```python
from build123d import *

# Parameters (mm, degrees)
SKETCH015_W                     = 86
SKETCH015_H                     = 175
PAD007_DEPTH                    = 40
SKETCH016_W                     = 84
SKETCH016_H                     = 173
POCKET007_DEPTH                 = 38
SKETCH017_W                     = 23
SKETCH017_H                     = 14
PAD008_DEPTH                    = 20
SKETCH017_LINEARPATTERN003_2_W  = 23
SKETCH017_LINEARPATTERN003_2_H  = 14
PAD008_LINEARPATTERN003_2_DEPTH = 20
SKETCH017_LINEARPATTERN003_3_W  = 23
SKETCH017_LINEARPATTERN003_3_H  = 14
PAD008_LINEARPATTERN003_3_DEPTH = 20
SKETCH017_LINEARPATTERN003_4_W  = 23
SKETCH017_LINEARPATTERN003_4_H  = 14
PAD008_LINEARPATTERN003_4_DEPTH = 20
SKETCH017_LINEARPATTERN003_5_W  = 23
SKETCH017_LINEARPATTERN003_5_H  = 14
PAD008_LINEARPATTERN003_5_DEPTH = 20
LINEARPATTERN004_COUNT          = 2
LINEARPATTERN004_PITCH          = 28
FILLET008_R                     = 5
FILLET009_R                     = 2


with BuildPart() as part:
    # Sketch015 → Pad007 (new body)
    with BuildSketch(Plane.XY):
        Rectangle(SKETCH015_W, SKETCH015_H)
    extrude(amount=PAD007_DEPTH)

    # Sketch016 (on DatumPlane) → Pocket007 (cut)
    with BuildSketch(Plane.XY.offset(40)):
        Rectangle(SKETCH016_W, SKETCH016_H)
    extrude(amount=-POCKET007_DEPTH, mode=Mode.SUBTRACT)

    # Sketch017 (on DatumPlane) → Pad008 (join)
    with BuildSketch(Plane(origin=(-20, 65, 2), x_dir=(1, 0, 0), z_dir=(0, 0, 1))):
        Rectangle(SKETCH017_W, SKETCH017_H)
    pad008 = extrude(amount=PAD008_DEPTH)

    # Sketch017 LinearPattern003 2 → Pad008 LinearPattern003 2 (add)
    with BuildSketch(Plane(origin=(-20, 32.5, 2), x_dir=(1, 0, 0), z_dir=(0, 0, 1))):
        Rectangle(SKETCH017_LINEARPATTERN003_2_W, SKETCH017_LINEARPATTERN003_2_H)
    pad008_linearpattern003_2 = extrude(amount=PAD008_LINEARPATTERN003_2_DEPTH)

    # Sketch017 LinearPattern003 3 → Pad008 LinearPattern003 3 (add)
    with BuildSketch(Plane(origin=(-20, 0, 2), x_dir=(1, 0, 0), z_dir=(0, 0, 1))):
        Rectangle(SKETCH017_LINEARPATTERN003_3_W, SKETCH017_LINEARPATTERN003_3_H)
    pad008_linearpattern003_3 = extrude(amount=PAD008_LINEARPATTERN003_3_DEPTH)

    # Sketch017 LinearPattern003 4 → Pad008 LinearPattern003 4 (add)
    with BuildSketch(Plane(origin=(-20, -32.5, 2), x_dir=(1, 0, 0), z_dir=(0, 0, 1))):
        Rectangle(SKETCH017_LINEARPATTERN003_4_W, SKETCH017_LINEARPATTERN003_4_H)
    pad008_linearpattern003_4 = extrude(amount=PAD008_LINEARPATTERN003_4_DEPTH)

    # Sketch017 LinearPattern003 5 → Pad008 LinearPattern003 5 (add)
    with BuildSketch(Plane(origin=(-20, -65, 2), x_dir=(1, 0, 0), z_dir=(0, 0, 1))):
        Rectangle(SKETCH017_LINEARPATTERN003_5_W, SKETCH017_LINEARPATTERN003_5_H)
    pad008_linearpattern003_5 = extrude(amount=PAD008_LINEARPATTERN003_5_DEPTH)

    # LinearPattern004: Pad008, Pad008 LinearPattern003 2, Pad008 LinearPattern003 3, Pad008 LinearPattern003 4, Pad008 LinearPattern003 5 ×2
    with Locations(*[(i * LINEARPATTERN004_PITCH, 0, 0) for i in range(1, LINEARPATTERN004_COUNT)]):
        add(pad008)
        add(pad008_linearpattern003_2)
        add(pad008_linearpattern003_3)
        add(pad008_linearpattern003_4)
        add(pad008_linearpattern003_5)

    # Fillet008
    fillet008_edges = [part.edges().sort_by_distance(p)[0] for p in [
        (-20, -25.5, 22),
        (-8.5, -32.5, 22),
        (-20, -39.5, 22),
        (-31.5, -32.5, 22),
        (-20, -58, 22),
        (-8.5, -65, 22),
        (-20, -72, 22),
        (-31.5, -65, 22),
        (8, -58, 22),
        (19.5, -65, 22),
        (8, -72, 22),
        (-3.5, -65, 22),
        (8, -25.5, 22),
        (19.5, -32.5, 22),
        (8, -39.5, 22),
        (-3.5, -32.5, 22),
        (-20, 7, 22),
        (-8.5, 0, 22),
        (-20, -7, 22),
        (-31.5, 0, 22),
        (8, 7, 22),
        (19.5, 0, 22),
        (8, -7, 22),
        (-3.5, 0, 22),
        (8, 39.5, 22),
        (19.5, 32.5, 22),
        (8, 25.5, 22),
        (-3.5, 32.5, 22),
        (-20, 72, 22),
        (-8.5, 65, 22),
        (-20, 58, 22),
        (-31.5, 65, 22),
        (8, 72, 22),
        (19.5, 65, 22),
        (8, 58, 22),
        (-3.5, 65, 22),
        (-20, 39.5, 22),
        (-8.5, 32.5, 22),
        (-20, 25.5, 22),
        (-31.5, 32.5, 22),
    ]]
    fillet(fillet008_edges, radius=FILLET008_R)

    # Fillet009
    fillet009_edges = [part.edges().sort_by_distance(p)[0] for p in [
        (0, 87.5, 0),
        (43, 0, 0),
        (0, -87.5, 0),
        (-43, 0, 0),
    ]]
    fillet(fillet009_edges, radius=FILLET009_R)


with BuildPart() as part_1:
    # Body006 placement: moved
    add(part.part.moved(Location((-51, -51, 0))))


solid = part_1.part
```
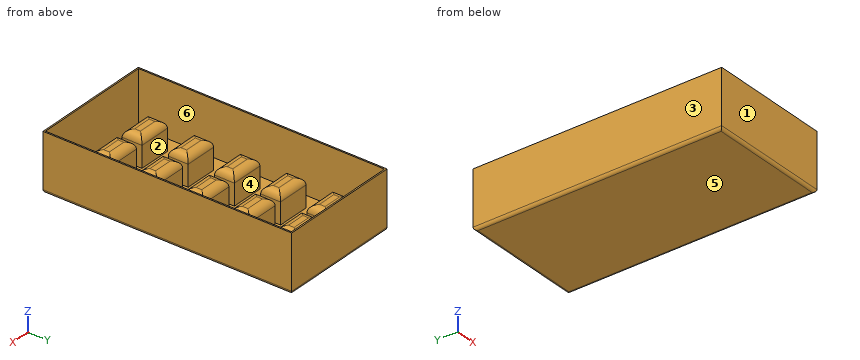
Check sheet for the modelled part. Datum: model origin and axes. Units: mm. Face numbers are marked on the shaded views. A direction names the side the tool comes from. Give positions to 0.01 mm unless a question says otherwise; leave off trailing zeros. Write each loop counter-clockwise with the first axis right and the second up, starting at its lowest first coordinate (ties: lowest second). Pieces come first, ordered by that corner, then holes.
Item 1: Draft check along X on the marked faces 3, 4, 5 and 6. Enter one of: released by +X, released by -X, zero draft, split by the parting line, or undercut.
Item 2: Scan lines: L1, parallel to X at y = -85, z = 37.5; L2, parallel to Y at x = -29, z = 31.5; L3, parallel to Z at x = -33.5, y = -126. Record each from-to range of solid material in increasing order.
Item 3: Cross-section at D-D (z = 35). Enter the section's corners in (x, y).
Item 4: Cross-section at A-A (z = 7.5). Count the separate pieces of the cut face and the enclosed holes in it, and give its area (3 significant figures).
Item 5: Cross-section at B-B (y = -99). Enter the section's corners in (x, z), and give its area (3 significant figures).
Item 6: Gauge pin test, flat ends, axial feed: pin 1 (4.5 mm diameter, centred on x = -40, y = -116.5, fed in from +Z); pin 2 (3 mm diameter, centred on x = -60, y = -49.5, fed in from +Z). Record the tip position at first contact, or that the pin passes through.
Item 7: Access from +Z, -Z, +X, -X, +Y, -Y to the whole of each face (thin tool, end or side, straight path). Record for the marked faces 1 and 2.
Item 8: Cross-section at C-C (x = -14). Enter the section's corners in (y, z), and give its area (3 significant figures).
Report:
1. face 3: released by -X
1. face 4: undercut
1. face 5: zero draft
1. face 6: undercut
2. L1: x = -94 to -93, -9 to -8
2. L2: y = -138.5 to -137.5, 35.5 to 36.5
2. L3: z = 0 to 2
3. outline: (-94, -138.5) - (-8, -138.5) - (-8, 36.5) - (-94, 36.5) - close; hole (-93, -137.5) - (-9, -137.5) - (-9, 35.5) - (-93, 35.5) - close
4. separate pieces: 11
4. enclosed holes: 1
4. area: 3,740 mm2
5. outline: (-94, 2) arc R2 ccw to (-92, 0) - (-10, 0) arc R2 ccw to (-8, 2) - (-8, 40) - (-9, 40) - (-9, 2) - (-93, 2) - (-93, 40) - (-94, 40) - close
5. area: 246 mm2
6. pin 1: stops at z = 22
6. pin 2: stops at z = 21
7. face 1: +Z, -Z, +X, -X, -Y
7. face 2: +Z
8. outline: (-138.5, 2) arc R2 ccw to (-136.5, 0) - (34.5, 0) arc R2 ccw to (36.5, 2) - (36.5, 40) - (35.5, 40) - (35.5, 2) - (-137.5, 2) - (-137.5, 40) - (-138.5, 40) - close
8. area: 424 mm2
